Part model, mm, in its own coordinate system. Round coordinates to 2 decimals unless told otherwise and drop trailing zeros. Write each loop counter-clockwise with the first axis right and the second up, starting at its lowest first coordinate (ties: lowest second). Pieces come first, ordered by that corner, then holes.
from build123d import *

# Parameters (mm, degrees)
SKETCH1_R                      = 25.4
BOSS_EXTRUDE1_DEPTH            = 38.1
F_1_4_20_TAPPED_HOLE4_D        = 5.1054
F_1_4_20_TAPPED_HOLE4_DEPTH    = 15.875
F_1_4_20_TAPPED_HOLE4_TIP      = 1.533816902
CBORE_FOR_M3_SHCS1_D           = 3.2
CBORE_FOR_M3_SHCS1_CBORE_D     = 6.5
CBORE_FOR_M3_SHCS1_CBORE_DEPTH = 4.999996


with BuildPart() as part:
    # Sketch1 → Boss-Extrude1 (new body)
    with BuildSketch(Plane(origin=(0, 0, 0), x_dir=(1, 0, 0), z_dir=(0, 1, 0))):
        with Locations(Location((0, 0, 0), (0, 0, 90))):
            Circle(SKETCH1_R)
    extrude(amount=BOSS_EXTRUDE1_DEPTH)

    # 1_4-20 Tapped Hole4
    with Locations(Plane(origin=(0, 0, 0), x_dir=(-1, 0, 0), z_dir=(0, -1, 0))):
        with Locations((12.7, 0), (-12.7, 0)):
            Hole(F_1_4_20_TAPPED_HOLE4_D / 2, depth=F_1_4_20_TAPPED_HOLE4_DEPTH)
            with Locations((0, 0, -(F_1_4_20_TAPPED_HOLE4_DEPTH + F_1_4_20_TAPPED_HOLE4_TIP / 2))):  # 118° drill point
                Cone(0, F_1_4_20_TAPPED_HOLE4_D / 2, F_1_4_20_TAPPED_HOLE4_TIP, mode=Mode.SUBTRACT)

    # CBORE for M3 SHCS1 (through all)
    with Locations(Plane(origin=(0, 0, 0), x_dir=(-1, 0, 0), z_dir=(0, -1, 0))):
        with Locations((0, -12.7), (0, 12.7)):
            CounterBoreHole(CBORE_FOR_M3_SHCS1_D / 2, CBORE_FOR_M3_SHCS1_CBORE_D / 2, CBORE_FOR_M3_SHCS1_CBORE_DEPTH)


solid = part.part
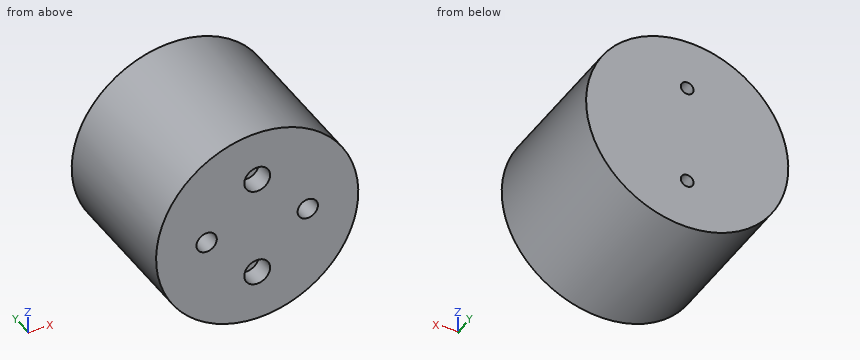
Q1. Drop flat-ended pins along their axis: P1, Ø2, axis at y = 13.5, z = 10.5, coming from the -X side; P2, Ø4, axis at y = 29.5, z = 2.5, coming from the -X side; P3, Ø6, axis at y = 6, z = -4.5, coming from the +X side; P4, Ø2.5, axis at x = 0, z = -12.7, coming from the +Y side. Give the stop position or say it passes through.
Q2. Saw through at C-C, the plane y = 23. Write the cut outline in (x, z), and give its area (3 significant figures).
Q3. Wall check: line 1 (Z direction, x = 0.5, y = 12); line 2 (X direction, y = 16, z = -12); line 3 (X direction, y = 13.5, z = 1.5). Give the ranges that are in metal, low to high.
Q4. Saw through at D-D, the plane z = -17.5. Write the cut outline in (x, y), and give its area (3 significant figures).
Q5. Saw through at B-B, the plane z = 12.7. Write the cut outline in (x, y).
Q6. Saw through at A-A, the plane y = 11.5. Write the cut outline in (x, z).
Computed:
1. P1: stops at x = -23.56
1. P2: stops at x = -25.4
1. P3: stops at x = 25.36
1. P4: passes through
2. outline: circle Ø50.8 at (0, 0); hole circle Ø3.2 at (0, -12.7); hole circle Ø3.2 at (0, 12.7)
2. area: 2,010 mm2
3. line 1: z = -25.4 to -14.22, -11.18 to 11.18, 14.22 to 25.4
3. line 2: x = -22.39 to -1.44, 1.44 to 22.39
3. line 3: x = -25.36 to -14.77, -10.63 to 10.63, 14.77 to 25.36
4. outline: (-18.41, 0) - (18.41, 0) - (18.41, 38.1) - (-18.41, 38.1) - close
4. area: 1,400 mm2
5. outline: (-22, 0) - (-3.25, 0) - (-3.25, 5) - (-1.6, 5) - (-1.6, 38.1) - (-22, 38.1) - close; (1.6, 5) - (3.25, 5) - (3.25, 0) - (22, 0) - (22, 38.1) - (1.6, 38.1) - close
6. outline: circle Ø50.8 at (0, 0); hole circle Ø5.11 at (-12.7, 0); hole circle Ø3.2 at (0, -12.7); hole circle Ø3.2 at (0, 12.7); hole circle Ø5.11 at (12.7, 0)
